```python
from build123d import *

# Parameters (mm, degrees)
F0_W     = 65
F0_H     = 5
F1_DEPTH = 65
F2_R     = 2.75
F2_R_2   = 5
F3_DEPTH = 5


with BuildPart() as f1:
    # F0 (on Front) → F1 (new body)
    with BuildSketch(Plane.XZ):
        with Locations((-32.5, 2.5)):
            Rectangle(F0_W, F0_H)
    extrude(amount=-F1_DEPTH)

    # F2 (on Top) → F3 (cut)
    with BuildSketch(Plane.XY):
        with Locations((-10, 48)):
            Circle(F2_R)
        with Locations((-10, 17)):
            Circle(F2_R)
        with Locations((-41, 51)):
            Circle(F2_R)
        with Locations((-41, 14)):
            Circle(F2_R)
        with Locations((-41, 32.5)):
            Circle(F2_R_2)
    extrude(amount=F3_DEPTH, mode=Mode.SUBTRACT)


solid = f1.part
```
Source: CAD feature listing. Evaluate the final solid. Frame: model axes, mm. Give positions to 0.01 mm unless a question says otherwise; leave off trailing zeros. Write each loop counter-clockwise with the first axis right and the second up, starting at its lowest first coordinate (ties: lowest second). Pieces come first, ordered by that corner, then holes.
1. Section query A-A (y = 32.5). Return the cut outline in (x, z).
2. First-contact query: pin 1 (5 mm diameter, centred on x = -41, y = 14, fed in from +Z). Flat tip, straight axial feed; report the tip coordinate or a pass-through.
3. Section query D-D (z = 3.35). Return the cut outline in (x, y).
4. Pull-direction query (X, two-part tool) for faces 1 (the face through (-65, 32, 2)), 2 (the face through (-45.995, 32.72, 2.465)), 3 (the face through (0, 32, 2)), 4 (the face through (-33, 32, 5)); classes: +X half, -X half, draft (parallel to the pull), parting line (faces both ways), or undercut.
5. Section query C-C (x = -10). Return the cut outline in (y, z).
6. Section query B-B (x = -41). Return the cut outline in (y, z), then the cut area to 3 significant figures.
7. Material intervals for line 1 along Y through (x, z) = (-41, 1.1); line 2 along Y through (x, z) = (-10, 2.05); line 3 along X through (y, z) = (50.5, 3.45), sorted ascending.
Output values:
1. outline: (-65, 0) - (-46, 0) - (-46, 5) - (-65, 5) - close; (-36, 0) - (0, 0) - (0, 5) - (-36, 5) - close
2. pin 1: passes through
3. outline: (-65, 0) - (0, 0) - (0, 65) - (-65, 65) - close; hole circle Ø10 at (-41, 32.5); hole circle Ø5.5 at (-41, 14); hole circle Ø5.5 at (-41, 51); hole circle Ø5.5 at (-10, 17); hole circle Ø5.5 at (-10, 48)
4. face 1: -X half
4. face 2: undercut
4. face 3: +X half
4. face 4: draft
5. outline: (0, 0) - (14.25, 0) - (14.25, 5) - (0, 5) - close; (19.75, 0) - (45.25, 0) - (45.25, 5) - (19.75, 5) - close; (50.75, 0) - (65, 0) - (65, 5) - (50.75, 5) - close
6. outline: (0, 0) - (11.25, 0) - (11.25, 5) - (0, 5) - close; (16.75, 0) - (27.5, 0) - (27.5, 5) - (16.75, 5) - close; (37.5, 0) - (48.25, 0) - (48.25, 5) - (37.5, 5) - close; (53.75, 0) - (65, 0) - (65, 5) - (53.75, 5) - close
6. area: 220 mm2
7. line 1: y = 0 to 11.25, 16.75 to 27.5, 37.5 to 48.25, 53.75 to 65
7. line 2: y = 0 to 14.25, 19.75 to 45.25, 50.75 to 65
7. line 3: x = -65 to -43.7, -38.3 to -11.15, -8.85 to 0
